```python
from build123d import *

# Parameters (mm, degrees)
F0_W     = 175
F0_H     = 20
F0_W_2   = 150
F0_H_2   = 80
F1_DEPTH = 20
F2_W     = 150
F2_H     = 80
F2_H_2   = 20
F3_DEPTH = 10


with BuildPart() as f1:
    # F0 (on Top) → F1 (new body)
    with BuildSketch(Plane.XY):
        with Locations((-162.5, 50)):
            Rectangle(F0_W, F0_H)
        with Locations((162.5, 50)):
            Rectangle(F0_W, F0_H)
        with Locations((-162.5, -50)):
            Rectangle(F0_W, F0_H)
        with Locations((162.5, -50)):
            Rectangle(F0_W, F0_H)
        Rectangle(F0_W_2, F0_H_2)
        with Locations((0, -50)):
            Rectangle(F0_W_2, F0_H)
        with Locations((0, 50)):
            Rectangle(F0_W_2, F0_H)
    extrude(amount=F1_DEPTH)

    # F2 (on face) → F3 (join)
    with BuildSketch(Plane.XY.offset(20)):
        Rectangle(F2_W, F2_H)
        with Locations((0, 50)):
            Rectangle(F2_W, F2_H_2)
        with Locations((0, -50)):
            Rectangle(F2_W, F2_H_2)
    extrude(amount=F3_DEPTH)


solid = f1.part
```
Verification items for the finished model (mm, model axes). A direction names the side the tool comes from. Give positions to 0.01 mm unless a question says otherwise; leave off trailing zeros. Order: outer loops, then holes, each group sorted by start corner. A loop starts at its lowest first (then second) coordinate and runs counter-clockwise, first axis right, second up. Notation, with made-up numbers: M 29,81 L 76,81 A9 ccw 76,95 Z; hole C 31,38.25 d9. An arc over 180 degrees is marked long. Return JSON: item names as keys, results as strings. Group by question number.
1) Access from +Z, -Z, +X, -X, +Y, -Y to the whole of each face (thin tool, end or side, straight path). Record for faces 4 (the face through (161, 40, 10)), 5 (the face through (-164, 50, 20)), 6 (the face through (-164, -40, 10)), 7 (the face through (161, -50, 20)).
2) Section check C-C on z = 9.75. Record the cut outline in (x, y), and give its area (3 significant figures).
3) Mould release check, pull along Y, two halves, no side actions. Record for faces 1 (the face through (75, -1, 15)), 2 (the face through (-3, 60, 11)), 3 (the face through (161, 50, 20)): pulls with the +Y half, pulls with the -Y half, needs draft (parallel to the pull), parting line crosses it, or undercut.
4) Section check A-A on x = -163. Record the cut outline in (y, z).
5) Section check B-B on y = 45.5. Record the cut outline in (x, z).
6) Go/stop test with flat-tipped pins: pin 1 Ø1 at (y, z) = (13.5, 12) entering from +X; pin 2 Ø1.5 at (y, z) = (-38, 4) entering from -X; pin 3 Ø22 at (x, y) = (150.5, 52.5) entering from +Z. Record where each tip stops, or that it passes through.
7) Scan lines: line 1 (Y direction, x = 214.5, z = 9.75); line 2 (Z direction, x = -89, y = -44.5); line 3 (X direction, y = 23.5, z = 25.25). Record each from-to range of solid material in increasing order.
Answer block:
{
 "1": {"face 4": "+Z, -Z, +X", "face 5": "+Z, -X, +Y, -Y", "face 6": "+Z, -Z, -X", "face 7": "+Z, +X, +Y, -Y"},
 "2": {"outline": "M -250,-60 L 250,-60 L 250,-40 L 75,-40 L 75,40 L 250,40 L 250,60 L -250,60 L -250,40 L -75,40 L -75,-40 L -250,-40 Z", "area": "32,000 mm^2"},
 "3": {"face 1": "undercut", "face 2": "pulls with the +Y half", "face 3": "needs draft"},
 "4": {"outline": "M -60,0 L -40,0 L -40,20 L -60,20 Z; M 40,0 L 60,0 L 60,20 L 40,20 Z"},
 "5": {"outline": "M -250,0 L 250,0 L 250,20 L 75,20 L 75,30 L -75,30 L -75,20 L -250,20 Z"},
 "6": {"pin 1": "stops at x = 75", "pin 2": "stops at x = -75", "pin 3": "stops at z = 20"},
 "7": {"line 1": "y = -60 to -40, 40 to 60", "line 2": "z = 0 to 20", "line 3": "x = -75 to 75"}
}
